Here's how the part is built. I have some questions about the finished solid (model axes, mm). Face numbers are marked on the shaded views. A direction names the side the tool comes from. Round coordinates to 2 decimals unless told otherwise and drop trailing zeros. Order: outer loops, then holes, each group sorted by start corner. A loop starts at its lowest first (then second) coordinate and runs counter-clockwise, first axis right, second up. Notation, with made-up numbers: (-21.5, -1.5) - (-8.5, -1.5) arc R27 cw to (-8.5, 17.5) - close; hole circle Ø11 at (67, -34). An arc over 180 degrees is marked (long way). One line per item, written item: value.
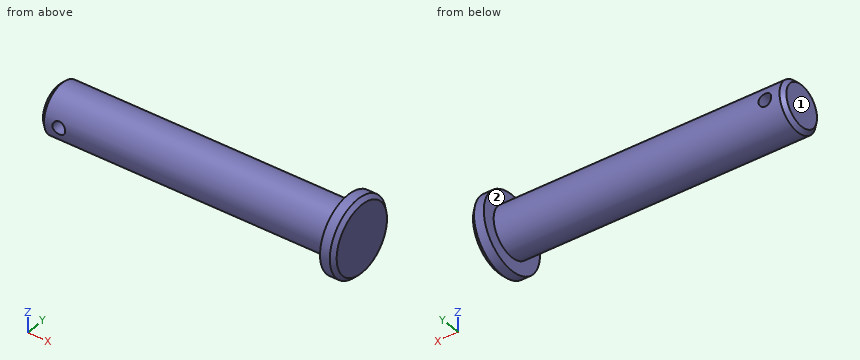
from build123d import *

# Parameters (mm, degrees)
CORTE_EXTRUS_O1_DEPTH      = 82.967885327
CORTE_EXTRUS_O1_DEPTH_BACK = 82.967885327
ESBO_O2_R                  = 3.25


with BuildPart() as part:
    # Esboço1 → Revolução1 (revolve)
    with BuildSketch(Plane.XY, mode=Mode.PRIVATE) as revolu_o1_sk:
        Polygon((77.315, 0), (77.315, 17.25), (75.315, 19.25), (70.315, 19.25), (70.315, 12.5), (-75.315, 12.5), (-77.315, 10.5), (-77.315, 0), align=None)
    revolve(revolu_o1_sk.sketch.rotate(Axis((-77.315, 0, 0), (1, 0, 0)), 90), axis=Axis((-77.315, 0, 0), (1, 0, 0)))

    # Esboço2 → Corte-extrusão1 (cut, two sides: drawn at the far end of the back side and taken through both)
    with BuildSketch(Plane(origin=(0, 0, 0), x_dir=(1, 0, 0), z_dir=(0, 1, 0)).offset(-CORTE_EXTRUS_O1_DEPTH_BACK)):
        with Locations(Location((-67.815, 0, 0), (0, 0, 270))):
            Circle(ESBO_O2_R)
    extrude(amount=CORTE_EXTRUS_O1_DEPTH + CORTE_EXTRUS_O1_DEPTH_BACK, mode=Mode.SUBTRACT)


solid = part.part
Q1. If we section it at A-A, the plane z = 0: Please give me the cut outline in (x, y) (3 decimals).
Results list:
outline: (-77.315, -10.5) - (-75.315, -12.5) - (-71.065, -12.5) - (-71.065, 12.5) - (-75.315, 12.5) - (-77.315, 10.5) - close; (-64.565, -12.5) - (70.315, -12.5) - (70.315, -19.25) - (75.315, -19.25) - (77.315, -17.25) - (77.315, 17.25) - (75.315, 19.25) - (70.315, 19.25) - (70.315, 12.5) - (-64.565, 12.5) - close
Q2. Which directions (+Z, -Z, +X, -X, +Y, -Y) give clear straight access to the entire face, cutting with the end or side of a thin tool? Please do the marked faces 1 and 2.
Results list:
face 1: +Z, -Z, -X, +Y, -Y
face 2: -X
Q3. Will these pins go through, and if not, where does the flat tip stop? pin 1 (3 mm diameter, centred on x = -12.5, y = -6.5, fed in from +Z); pin 2 (10 mm diameter, centred on x = 6.5, y = 5.5, fed in from -Z); pin 3 (4 mm diameter, centred on x = 19.5, y = 10.5, fed in from +Z).
Results list:
pin 1: z = 11.46
pin 2: z = -12.49
pin 3: z = 9.17
Q4. If we section it at B-B, the plane y = 0: Please give me the cut outline in (x, z) (3 decimals), then the cut area to 3 significant figures.
Results list:
outline: (-77.315, -10.5) - (-75.315, -12.5) - (70.315, -12.5) - (70.315, -19.25) - (75.315, -19.25) - (77.315, -17.25) - (77.315, 17.25) - (75.315, 19.25) - (70.315, 19.25) - (70.315, 12.5) - (-75.315, 12.5) - (-77.315, 10.5) - close; hole circle Ø6.5 at (-67.815, 0)
area: 3,920 mm²
Q5. If we section it at C-C, the plane x = 39: Please give me the cut outline in (y, z).
Results list:
outline: circle Ø25 at (0, 0)
Q6. If I drill on line 1 along X through (y, z) = (-7, 0) (3 decimals); line 2 along X through (y, z) = (17, -1) (3 decimals); line 3 along Z through (x, y) = (-65.5, 4), over which ranges is the centre line in solid material (lowest first)?
Results list:
line 1: -77.315 to -71.065, -64.565 to 77.315
line 2: 70.315 to 77.315
line 3: -11.84 to -2.28, 2.28 to 11.84
